Model file for the job. Use its own axes, mm. Face numbers are marked on the shaded views. A direction names the side the tool comes from. Round coordinates to 2 decimals unless told otherwise and drop trailing zeros. Loops run counter-clockwise (first coordinate to the right, second up) from the corner with the lowest first, then second, coordinate; pieces in that order, holes last. Notation, with made-up numbers: M -2,68 L 46,68 A14 cw 46,85 Z; hole C 80,78 d4. An arc over 180 degrees is marked long. Use a Markdown table: item, result. Add a question column.
Q1. Cut at A-A (y = 69). Give the cut face in (x, z), plus the area to 3 significant figures.
Q2. Tool access for the marked faces 1 and 2: list every direction of +Z, -Z, +X, -X, +Y, -Y with a clear straight run to the whole face (end or side of a thin tool).
Q3. Cut at B-B (x = -84.5). Give the cut face in (y, z), plus the area to 3 significant figures.
Q4. Probe line 1 (Z direction, x = -134, y = 66); line 2 (Y direction, x = -134.3, z = 12.7); line 3 (Y direction, x = -26, z = 18.5). List the from-to ranges inside material, lowest first. Write a range as from..to.
Q5. Cut at C-C (y = 42.5). Give the cut face in (x, z).
Q6. Pin check, flat tips, straight feed: pin 1 (1.3 mm diameter, centred on y = 1, z = 10, fed in from +X); pin 2 (0.5 mm diameter, centred on x = -10, z = 1, fed in from -Y); pin 3 (1.7 mm diameter, centred on x = -1, z = 8.5, fed in from +Y); pin 4 (1.3 mm diameter, centred on y = 25, z = 11.5, fed in from +X). Stop position of each tip, or through.
Q7. Cut at D-D (z = 12.7). State how many separate pieces and enclosed holes the cut face has, plus the area to 3 significant figures.
from build123d import *

# Parameters (mm, degrees)
BOSS_EXTRUDE1_DEPTH      = 1.5875
SKETCH2_W                = 1.5875
SKETCH2_H                = 1.5875
BOSS_EXTRUDE2_DEPTH      = 132.842
SKETCH3_W                = 25.4
SKETCH3_H                = 25.4
SKETCH3_W_2              = 22.225
SKETCH3_H_2              = 22.225
BOSS_EXTRUDE3_DEPTH      = 1.5875
BOSS_EXTRUDE4_START      = -1.5875
BOSS_EXTRUDE4_DEPTH      = 22.225
BOSS_EXTRUDE5_DEPTH      = 1.5875
LPATTERN1_COUNT          = 5
LPATTERN1_PITCH          = 26.162
MIRROR6_COPY_1_DEPTH     = 1.5875
MIRROR6_COPY_2_DEPTH     = 1.5875
MIRROR6_COPY_3_DEPTH     = 1.5875
MIRROR6_COPY_4_DEPTH     = 1.5875
BOSS_EXTRUDE6_START      = -1.5875
SKETCH10_W               = 1.5875
SKETCH10_H               = 1.5875
BOSS_EXTRUDE6_DEPTH      = 22.225
LPATTERN2_COUNT          = 5
LPATTERN2_PITCH          = 26.162
SKETCH12_W               = 25.4
SKETCH12_H               = 17.4625
BOSS_EXTRUDE13_DEPTH     = 1.5875
M3_CLEARANCE_HOLE1_D     = 3.4
M3_CLEARANCE_HOLE1_DEPTH = 1.5875
SKETCH19_W               = 3.175
SKETCH19_H               = 25.4
BOSS_EXTRUDE14_DEPTH     = 66.04
BOSS_EXTRUDE15_DEPTH     = 3.175
SKETCH21_R               = 6.35
CUT_EXTRUDE1_DEPTH       = 3.175


with BuildPart() as part:
    # Sketch1 → Boss-Extrude1 (new body)
    with BuildSketch(Plane.XY):
        Polygon((0, 0), (0, 25.4), (9.525, 8.902216058), align=None)
        Polygon((7.519534439, 9.200784302), (1.5875, 3.656610839), (1.5875, 19.475369343), align=None, mode=Mode.SUBTRACT)
    extrude(amount=BOSS_EXTRUDE1_DEPTH)

    # Sketch2 → Boss-Extrude2 (add)
    with BuildSketch(Plane.ZY):
        with Locations((0.79375, 24.60625)):
            Rectangle(SKETCH2_W, SKETCH2_H)
        with Locations((0.79375, 0.79375)):
            Rectangle(SKETCH2_W, SKETCH2_H)
    extrude(amount=BOSS_EXTRUDE2_DEPTH)

    # Sketch3 → Boss-Extrude3 (add)
    with BuildSketch(Plane.ZY.offset(132.842)):
        with Locations((12.7, 12.7)):
            Rectangle(SKETCH3_W, SKETCH3_H)
        with Locations((12.7, 12.7)):
            Rectangle(SKETCH3_W_2, SKETCH3_H_2, mode=Mode.SUBTRACT)
    boss_extrude3 = extrude(amount=-BOSS_EXTRUDE3_DEPTH)

    # Mirror4: part across plane


with BuildPart() as part_1:
    add(part.part)
    add(part.part.mirror(Plane.XY.offset(12.7)))

    # Mirror5: Boss-Extrude3 across plane
    add(boss_extrude3.mirror(Plane(origin=(-66.421, 0, 0), x_dir=(0, 0, 1), z_dir=(1, 0, 0))))

    # Sketch7 → Boss-Extrude4 (add)
    with BuildSketch(Plane(origin=(0, 0, 0), x_dir=(-1, 0, 0), z_dir=(0, 0, -1)).offset(BOSS_EXTRUDE4_START)):
        Polygon((-9.525, 8.902216058), (-8.334375, 7.789439051), (-7.519534439, 9.200784302), (-8.710159439, 10.313561309), align=None)
    extrude(amount=-BOSS_EXTRUDE4_DEPTH)

    # Sketch9 → Boss-Extrude5 (add)
    with BuildSketch(Plane(origin=(0, 0, 0), x_dir=(-1, 0, 0), z_dir=(0, 0, -1))):
        Polygon((1.5875, 23.8125), (13.157102699, 1.5875), (14.744602699, 1.5875), (26.314205397, 23.8125), (24.726705397, 23.8125), (13.950852699, 3.112279563), (3.175, 23.8125), align=None)
    boss_extrude5 = extrude(amount=-BOSS_EXTRUDE5_DEPTH)

    # LPattern1: Boss-Extrude5 ×5
    with Locations(*[(-i * LPATTERN1_PITCH, 0, 0) for i in range(1, LPATTERN1_COUNT)]):
        add(boss_extrude5)

    # Mirror6: Boss-Extrude5 across plane
    add(boss_extrude5.mirror(Plane.XY.offset(12.7)))

    # Mirror6 copy 1 sketch → Mirror6 copy 1 (add)
    with BuildSketch(Plane(origin=(-26.162, 0, 25.4), x_dir=(-1, 0, 0), z_dir=(0, 0, 1))):
        Polygon((1.5875, -23.8125), (13.157102699, -1.5875), (14.744602699, -1.5875), (26.314205397, -23.8125), (24.726705397, -23.8125), (13.950852699, -3.112279563), (3.175, -23.8125), align=None)
    extrude(amount=-MIRROR6_COPY_1_DEPTH)

    # Mirror6 copy 2 sketch → Mirror6 copy 2 (add)
    with BuildSketch(Plane(origin=(-52.324, 0, 25.4), x_dir=(-1, 0, 0), z_dir=(0, 0, 1))):
        Polygon((1.5875, -23.8125), (13.157102699, -1.5875), (14.744602699, -1.5875), (26.314205397, -23.8125), (24.726705397, -23.8125), (13.950852699, -3.112279563), (3.175, -23.8125), align=None)
    extrude(amount=-MIRROR6_COPY_2_DEPTH)

    # Mirror6 copy 3 sketch → Mirror6 copy 3 (add)
    with BuildSketch(Plane(origin=(-78.486, 0, 25.4), x_dir=(-1, 0, 0), z_dir=(0, 0, 1))):
        Polygon((1.5875, -23.8125), (13.157102699, -1.5875), (14.744602699, -1.5875), (26.314205397, -23.8125), (24.726705397, -23.8125), (13.950852699, -3.112279563), (3.175, -23.8125), align=None)
    extrude(amount=-MIRROR6_COPY_3_DEPTH)

    # Mirror6 copy 4 sketch → Mirror6 copy 4 (add)
    with BuildSketch(Plane(origin=(-104.648, 0, 25.4), x_dir=(-1, 0, 0), z_dir=(0, 0, 1))):
        Polygon((1.5875, -23.8125), (13.157102699, -1.5875), (14.744602699, -1.5875), (26.314205397, -23.8125), (24.726705397, -23.8125), (13.950852699, -3.112279563), (3.175, -23.8125), align=None)
    extrude(amount=-MIRROR6_COPY_4_DEPTH)

    # Sketch10 → Boss-Extrude6 (add)
    with BuildSketch(Plane(origin=(0, 0, 0), x_dir=(-1, 0, 0), z_dir=(0, 0, -1)).offset(BOSS_EXTRUDE6_START)):
        with Locations((118.598852699, 0.79375)):
            Rectangle(SKETCH10_W, SKETCH10_H)
        with Locations((130.168455397, 24.60625)):
            Rectangle(SKETCH10_W, SKETCH10_H)
        with Locations((107.02925, 24.60625)):
            Rectangle(SKETCH10_W, SKETCH10_H)
    boss_extrude6 = extrude(amount=-BOSS_EXTRUDE6_DEPTH)

    # LPattern2: Boss-Extrude6 ×5
    with Locations(*[(i * LPATTERN2_PITCH, 0, 0) for i in range(1, LPATTERN2_COUNT)]):
        add(boss_extrude6)

    # Sketch12 → Boss-Extrude13 (add)
    with BuildSketch(Plane(origin=(10.998522628, 6.35, 0), x_dir=(0, 0, -1), z_dir=(0.8660254037844415, 0.49999999999999506, 0))):
        with Locations((-12.7, 11.678295256)):
            Rectangle(SKETCH12_W, SKETCH12_H)
    extrude(amount=BOSS_EXTRUDE13_DEPTH)

    # M3 Clearance Hole1
    with Locations(Plane(origin=(12.373337957, 7.14375, 0), x_dir=(0, 0, -1), z_dir=(0.8660254037844414, 0.49999999999999517, 0))):
        with Locations((-20.32, 15.329545256), (-20.32, 8.027045256), (-5.08, 15.329545256), (-5.08, 8.027045256)):
            Hole(M3_CLEARANCE_HOLE1_D / 2, depth=M3_CLEARANCE_HOLE1_DEPTH)

    # Sketch19 → Boss-Extrude14 (add)
    with BuildSketch(Plane(origin=(0, 0, 0), x_dir=(1, 0, 0), z_dir=(0, 1, 0))):
        with Locations((-134.4295, -12.7)):
            Rectangle(SKETCH19_W, SKETCH19_H)
    extrude(amount=BOSS_EXTRUDE14_DEPTH)

    # Sketch20 → Boss-Extrude15 (add)
    with BuildSketch(Plane.ZY.offset(136.017)):
        with BuildLine():
            Line((0, 66.04), (25.4, 66.04))
            ThreePointArc((25.4, 66.04), (12.7, 78.74), (0, 66.04))
        make_face()
    extrude(amount=-BOSS_EXTRUDE15_DEPTH)

    # Sketch21 → Cut-Extrude1 (cut)
    with BuildSketch(Plane.ZY.offset(136.017)):
        with Locations((12.7, 66.04)):
            Circle(SKETCH21_R)
        Polygon((1.5875, 29.718299952), (21.998939404, 52.3875), (1.5875, 52.3875), align=None)
        Polygon((1.5875, 1.5875), (21.56743597, 1.5875), (1.5875, 21.56743597), align=None)
        Polygon((3.83256403, 23.8125), (23.8125, 23.8125), (23.8125, 3.83256403), align=None)
        Polygon((3.401060596, 26.9875), (23.8125, 26.9875), (23.8125, 49.656700048), align=None)
    extrude(amount=-CUT_EXTRUDE1_DEPTH, mode=Mode.SUBTRACT)


solid = part_1.part
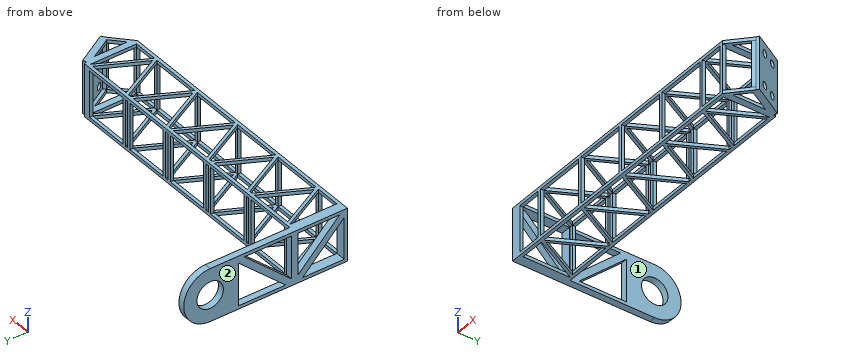
Checked values:
| question | item | result |
|---|---|---|
| 1 | outline | M -136.02,0.35 L -132.84,0.35 L -132.84,7.08 L -136.02,7.08 Z; M -136.02,18.32 L -132.84,18.32 L -132.84,25.05 L -136.02,25.05 Z |
| 1 | area | 42.8 mm^2 |
| 2 | face 1 | +Z, -Z, +X, +Y |
| 2 | face 2 | +Z, -Z, -X, +Y, -Y |
| 3 | outline | M 0,0 L 1.59,0 L 1.59,1.59 L 0,1.59 Z; M 0,23.81 L 1.59,23.81 L 1.59,25.4 L 0,25.4 Z; M 15.31,0 L 18.36,0 L 18.36,1.59 L 15.31,1.59 Z; M 15.31,23.81 L 18.36,23.81 L 18.36,25.4 L 15.31,25.4 Z; M 23.81,0 L 25.4,0 L 25.4,1.59 L 23.81,1.59 Z; M 23.81,23.81 L 25.4,23.81 L 25.4,25.4 L 23.81,25.4 Z |
| 3 | area | 19.8 mm^2 |
| 4 | line 1 | z = 0..6.35, 19.05..25.4 |
| 4 | line 2 | y = 0..1.59, 10.45..14.95, 23.81..26.99, 37.32..42.06, 52.39..59.69, 72.39..78.74 |
| 4 | line 3 | y = 23.81..25.4 |
| 5 | outline | M -136.02,0 L -132.84,0 L -132.84,1.59 L -136.02,1.59 Z; M -136.02,13.1 L -132.84,13.1 L -132.84,17.37 L -136.02,17.37 Z; M -136.02,23.81 L -132.84,23.81 L -132.84,25.4 L -136.02,25.4 Z |
| 6 | pin 1 | stops at x = 0 |
| 6 | pin 2 | stops at y = 0 |
| 6 | pin 3 | stops at y = 25.4 |
| 6 | pin 4 | stops at x = 2.44 |
| 7 | separate pieces | 23 |
| 7 | enclosed holes | 0 |
| 7 | area | 166 mm^2 |
